from build123d import *

# Parameters (mm, degrees)
LPATTERN1_COUNT = 6
LPATTERN1_PITCH = 6.477
FILLET1_R       = 1.5875


with BuildPart() as part:
    # Sketch2 → Revolve1 (revolve)
    with BuildSketch(Plane.XY):
        Polygon((25.4, 49.2125), (31.75, 49.2125), (31.75, 24.60625), (28.575, 24.60625), (28.575, 0), (22.225, 0), (22.225, 6.35), (23.8125, 6.35), (23.8125, 27.78125), (25.4, 27.78125), align=None)
    revolve(axis=Axis((0, -40.656569806, 0), (0, 1, 0)))

    # Sketch3 → Cut-Revolve1 (revolve, cut)
    with BuildSketch(Plane.XY):
        Polygon((31.75, 46.0375), (31.369, 42.799), (31.75, 39.5605), align=None)
        Polygon((28.575, 23.84425), (28.575, 17.36725), (28.194, 20.60575), align=None)
    cut_revolve1 = revolve(axis=Axis((0, -40.656569806, 0), (0, 1, 0)), mode=Mode.SUBTRACT)

    # LPattern1: Cut-Revolve1 ×6
    with Locations(*[(0, -i * LPATTERN1_PITCH, 0) for i in range(1, LPATTERN1_COUNT)]):
        add(cut_revolve1, mode=Mode.SUBTRACT)

    # Fillet1
    fillet1_edges = [part.edges().sort_by_distance(p)[0] for p in [
        (-31.514676471, 24.60625, 0),
    ]]
    fillet(fillet1_edges, radius=FILLET1_R)


solid = part.part
Could you check a few things on this model? Use its own coordinates, in mm. A direction names the side the tool comes from. Coordinates: 2 decimals unless noted, no trailing zeros. Order: outer loops, then holes, each group sorted by start corner. A loop starts at its lowest first (then second) coordinate and runs counter-clockwise, first axis right, second up. Notation, with made-up numbers: (78, -13) -> (125, -13) arc R15 cw to (125, 16) -> close; hole circle Ø11 at (30, 58.25). An arc over 180 degrees is marked (long way). One line per question, with ' | ' between items.
Q1. On a 3-axis mill with a long thin cutter (end or side, diameter ignored), from which of +Z, -Z, +X, -X, +Y, -Y can I reach the whole of each face in a straight line? I mean faces 4 (the face through (-28.547, 24.22, -1.256)), 5 (the face through (29.94, 42.96, -9.43)), 6 (the face through (20, 6.35, -11)). Say none if no direction works.
Return value:
face 4: -Y | face 5: none | face 6: +Y
Q2. Imagine slicing it at B-B on y = 15. Please give me the cut outline in (x, z) (1 decimal), and give its area (3 significant figures).
Return value:
outline: circle Ø56.6 at (0, 0); hole circle Ø47.6 at (0, 0) | area: 734 mm²
Q3. If I drill on L1, parallel to Y at x = 1, z = 23.5; L2, parallel to Y at x = -23.5, z = 17; L3, parallel to Z at x = -19, y = 17.5, over which ranges is the centre line in solid material (lowest first)?
Return value:
L1: 0 to 6.35 | L2: 24.61 to 49.21 | L3: -21.32 to -14.35, 14.35 to 21.32
Q4. Imagine slicing it at A-A on y = 31.5. Please give me the cut outline in (x, z), and give its area (3 significant figures).
Return value:
outline: circle Ø63.13 at (0, 0); hole circle Ø50.8 at (0, 0) | area: 1,100 mm²
Q5. Thinking about a two-plate mould opening in Z: for faces 1 (the face through (29.943, 42.596, -9.43)), 2 (the face through (-18.897, 17.216, 14.49)), 3 (the face through (27, 24.606, 11)), which applies, pulls with the +Z half, pulls with the -Z half, needs draft (parallel to the pull), parting line crosses it, or undercut?
Return value:
face 1: parting line crosses it | face 2: undercut | face 3: needs draft
Q6. I'm going to push flat-ended pins straight in: P1, Ø5, axis at y = 26.5, z = -12.5, coming from the +X side; P2, Ø6, axis at y = 42.5, z = -5, coming from the -X side; P3, Ø10, axis at x = -6.5, z = -21.5, coming from the +Y side; P4, Ø1, axis at y = 17.5, z = -10, coming from the -X side. Where does each tip first touch, or does it pass through?
Return value:
P1: x = 30.13 | P2: x = -31.53 | P3: y = 49.21 | P4: x = -26.94
